For this review, take the finished solid that the model builds, in its own axes (mm). A direction names the side the tool comes from. Give positions to 0.01 mm unless a question says otherwise; leave off trailing zeros. Order: outer loops, then holes, each group sorted by start corner. A loop starts at its lowest first (then second) coordinate and runs counter-clockwise, first axis right, second up. Notation, with made-up numbers: (-35.75, 71) - (-7.75, 71) arc R26 ccw to (-7.75, 103) - close; hole circle Ø1 at (42.25, 35.5). An arc over 180 degrees is marked (long way). Use a Markdown table: item, result. Add a question column.
1) We need section C-C on z = 7.25. Write out the cut boundary in (x, y), then the cut area to 3 significant figures.
2) Wall thickness on L1, parallel to Y at x = 46, z = 1.5; L2, parallel to Y at x = 63, z = 25; L3, parallel to Z at x = 62, y = -47.25: over which ranges is each line inside the solid? List them lowest first.
3) We need section A-A on x = 50. Write out the cut boundary in (y, z), then the cut area to 3 significant figures.
4) We need section D-D on x = 45. Write out the cut boundary in (y, z).
5) Machinability: for faces 1 (the face through (63.72, -63.173, 28.574)), 2 (the face through (43, -43, 10)), 3 (the face through (59.7, -46.9, 5.1)), which of the approach directions +Z, -Z, +X, -X, +Y, -Y give a long, thin tool a straight path to every point of the face, cutting with its end or side? Answer none if there is none.
6) Clearance check with a flat-ended pin moving along its axis: P1, Ø5.5, axis at x = 44.22, z = 20, coming from the +Y side. State where the tip first meets the part, or that it passes through.
7) Mouldability with a two-part tool opening along X and no side actions: class faces 4 (the face through (27.28, -45.14, 4.93)), 5 (the face through (44, -41.288, 5)), 6 (the face through (65.224, -61, 7)), 7 (the face through (45.353, -63.204, 21.771)) as released by +X, released by -X, zero draft, split by the parting line, or undercut.
8) We need section B-B on y = -59.75. Write out the cut boundary in (x, z), then the cut area to 3 significant figures.
```python
from build123d import *

# Parameters (mm, degrees)
F1_DEPTH = 10
F3_DEPTH = 25
F4_W     = 42
F4_H     = 2.2
F5_DEPTH = 20
F6_R     = 2.1
F7_DEPTH = 4
F8_R     = 5
F9_R     = 5


with BuildPart() as f1:
    # F0 (on Top) → F1 (new body)
    with BuildSketch(Plane.XY):
        with BuildLine():
            Line((51.723857, -41.288426), (36.723857, -41.288426))
            ThreePointArc((36.723857, -41.288426), (27.177916, -45.242484), (23.223857, -54.788426))
            Line((23.223857, -54.788426), (23.223857, -64.288426))
            Line((23.223857, -64.288426), (65.223857, -64.288426))
            Line((65.223857, -64.288426), (65.223857, -54.788426))
            ThreePointArc((65.223857, -54.788426), (61.269799, -45.242484), (51.723857, -41.288426))
        make_face()
    extrude(amount=F1_DEPTH)

    # F2 (on face) → F3 (cut)
    with BuildSketch(Plane.XY.offset(10)):
        with BuildLine():
            Line((51.523857, -43.488426), (36.723857, -43.488426))
            ThreePointArc((36.723857, -43.488426), (28.592129, -46.856698), (25.223857, -54.988426))
            Line((25.223857, -54.988426), (25.223857, -62.088426))
            Line((25.223857, -62.088426), (63.023857, -62.088426))
            Line((63.023857, -62.088426), (63.023857, -54.988426))
            ThreePointArc((63.023857, -54.988426), (59.655585, -46.856698), (51.523857, -43.488426))
        make_face()
    extrude(amount=-F3_DEPTH, mode=Mode.SUBTRACT)

    # F4 (on face) → F5 (join)
    with BuildSketch(Plane.XY.offset(10)):
        with Locations((44.223857, -63.188426)):
            Rectangle(F4_W, F4_H)
    extrude(amount=F5_DEPTH)

    # F6 (on face) → F7 (cut)
    with BuildSketch(Plane.XZ.offset(64.288426)):
        with Locations((44.223857, 20)):
            Circle(F6_R)
    extrude(amount=-F7_DEPTH, mode=Mode.SUBTRACT)

    # F8
    f8_edges = [f1.edges().sort_by_distance(p)[0] for p in [
        (65.223857, -63.188426, 30),
    ]]
    fillet(f8_edges, radius=F8_R)

    # F9
    f9_edges = [f1.edges().sort_by_distance(p)[0] for p in [
        (23.223857, -63.188426, 30),
    ]]
    fillet(f9_edges, radius=F9_R)


solid = f1.part
```
Checked values:
| question | item | result |
|---|---|---|
| 1 | outline | (23.22, -64.29) - (65.22, -64.29) - (65.22, -54.79) arc R13.5 ccw to (51.72, -41.29) - (36.72, -41.29) arc R13.5 ccw to (23.22, -54.79) - close; hole (25.22, -62.09) - (63.02, -62.09) - (63.02, -54.99) arc R11.5 ccw to (51.52, -43.49) - (36.72, -43.49) arc R11.5 ccw to (25.22, -54.99) - close |
| 1 | area | 241 mm² |
| 2 | L1 | -64.29 to -62.09, -43.49 to -41.29 |
| 2 | L2 | -64.29 to -62.09 |
| 2 | L3 | 0 to 10 |
| 3 | outline | (-64.29, 0) - (-62.09, 0) - (-62.09, 30) - (-64.29, 30) - close; (-43.49, 0) - (-41.29, 0) - (-41.29, 10) - (-43.49, 10) - close |
| 3 | area | 88.0 mm² |
| 4 | outline | (-64.29, 0) - (-62.09, 0) - (-62.09, 18.05) - (-64.29, 18.05) - close; (-64.29, 21.95) - (-62.09, 21.95) - (-62.09, 30) - (-64.29, 30) - close; (-43.49, 0) - (-41.29, 0) - (-41.29, 10) - (-43.49, 10) - close |
| 5 | face 1 | +Z, +X, +Y, -Y |
| 5 | face 2 | +Z, +X, -X, +Y |
| 5 | face 3 | +Z, -Z |
| 6 | P1 | y = -62.09 |
| 7 | face 4 | released by -X |
| 7 | face 5 | zero draft |
| 7 | face 6 | released by +X |
| 7 | face 7 | undercut |
| 8 | outline | (23.22, 0) - (25.22, 0) - (25.22, 10) - (23.22, 10) - close; (63.02, 0) - (65.22, 0) - (65.22, 10) - (63.02, 10) - close |
| 8 | area | 42.0 mm² |
